```python
from build123d import *

# Parameters (mm, degrees)
F0_W      = 116
F0_H      = 71
F0_W_2    = 70
F0_H_2    = 53
F1_DEPTH  = 2
F2_W      = 116
F2_H      = 71
F2_W_2    = 112
F2_H_2    = 66
F3_DEPTH  = 11
F4_R      = 2.5
F5_R      = 1
F6_R      = 4.5
F6_R_2    = 2
F7_DEPTH  = 5
F8_SIZE   = 1.99999
F9_W      = 15.5
F9_H      = 7.5
F9_W_2    = 26
F9_H_2    = 4
F10_DEPTH = 25
F11_DEPTH = 25


# Not quite as in the source:
# - a fillet or chamfer is up to 0.001 mm smaller than in the source, because OpenCascade refuses the exact size


with BuildPart() as f1:
    # F0 (on Top) → F1 (new body)
    with BuildSketch(Plane.XY):
        with Locations((58, 35.5)):
            Rectangle(F0_W, F0_H)
        with Locations((55, 35.5)):
            Rectangle(F0_W_2, F0_H_2, mode=Mode.SUBTRACT)
    extrude(amount=F1_DEPTH)

    # F2 (on face) → F3 (join)
    with BuildSketch(Plane.XY.offset(2)):
        with Locations((58, 35.5)):
            Rectangle(F2_W, F2_H)
        with Locations((58, 36)):
            Rectangle(F2_W_2, F2_H_2, mode=Mode.SUBTRACT)
    extrude(amount=F3_DEPTH)

    # F4
    f4_edges = [f1.edges().sort_by_distance(p)[0] for p in [
        (0, 0, 6.5),
        (116, 0, 6.5),
        (0, 71, 6.5),
        (116, 71, 6.5),
    ]]
    fillet(f4_edges, radius=F4_R)

    # F5
    f5_edges = [f1.edges().sort_by_distance(p)[0] for p in [
        (114, 3, 7.5),
        (2, 3, 7.5),
        (2, 69, 7.5),
        (114, 69, 7.5),
    ]]
    fillet(f5_edges, radius=F5_R)

    # F6 (on face) → F7 (join)
    with BuildSketch(Plane.XY.offset(2)):
        with Locations((7, 64)):
            Circle(F6_R)
        with Locations((7, 64)):
            Circle(F6_R_2, mode=Mode.SUBTRACT)
        with Locations((7, 8)):
            Circle(F6_R)
        with Locations((7, 8)):
            Circle(F6_R_2, mode=Mode.SUBTRACT)
        with Locations((109, 8)):
            Circle(F6_R)
        with Locations((109, 8)):
            Circle(F6_R_2, mode=Mode.SUBTRACT)
        with Locations((109, 64)):
            Circle(F6_R)
        with Locations((109, 64)):
            Circle(F6_R_2, mode=Mode.SUBTRACT)
    extrude(amount=F7_DEPTH)

    # F8 (size 2 in the source; OpenCascade refuses exactly that, so slightly less here)
    f8_edges = [f1.edges().sort_by_distance(p)[0] for p in [
        (90, 35.5, 0),
        (55, 9, 0),
        (20, 35.5, 0),
        (55, 62, 0),
    ]]
    chamfer(f8_edges, length=F8_SIZE)

    # F9 (on face) → F10 (cut)
    with BuildSketch(Plane(origin=(0, 0, 0), x_dir=(0, -1, 0), z_dir=(-1, 0, 0))):
        with Locations((-54.75, 12.75)):
            Rectangle(F9_W, F9_H)
        with Locations((-26, 11)):
            Rectangle(F9_W_2, F9_H_2)
    extrude(amount=-F10_DEPTH, mode=Mode.SUBTRACT)

    # F11 (cut): faces of the model
    f11_faces = [f1.faces().sort_by_distance(p)[0] for p in [
        (7, 8, 2),
        (7, 64, 2),
        (109, 8, 2),
        (109, 64, 2),
    ]]
    extrude(f11_faces, amount=-F11_DEPTH, mode=Mode.SUBTRACT)


solid = f1.part
```
Verification items for the finished model (mm, model axes). A direction names the side the tool comes from. Coordinates: 2 decimals unless noted, no trailing zeros. Loops run counter-clockwise (first coordinate to the right, second up) from the corner with the lowest first, then second, coordinate; pieces in that order, holes last. Notation, with made-up numbers: (26.25, 72.5) -> (53.25, 72.5) arc R7 cw to (53.25, 83.5) -> close; hole circle Ø5 at (48.5, 76.25). An arc over 180 degrees is marked (long way). Answer in a Markdown table with one row per item. Add a question column.
1. Material ranges on probe 1 along Y at (x, z) = (109, 1.2); probe 2 along Y at (x, z) = (109, 5.9); probe 3 along Y at (x, z) = (64.5, 10), recorded low to high. Write a range as [from, to].
2. Section check B-B, the plane z = 4.75. Give the number of separate pieces and of enclosed holes in the cut face, then the cut area to 3 significant figures.
3. Section check C-C, the plane z = 11.5. Enter the section's corners in (x, y).
4. Draft check along Y on faces 3 (the face through (6.41, 68.46, 4.46)), 4 (the face through (53, 1, 13)), 5 (the face through (57, 0, 6)). Enter one of: +Y half, -Y half, draft (parallel to the pull), parting line (faces both ways), or undercut.
5. Depth check by flat-ended pin: P1, Ø0.6, axis at x = 1, y = 23.5, coming from the +Z side; P2, Ø5, axis at x = 7, y = 64, coming from the +Z side; P3, Ø1.6, axis at x = 1, z = 10.5, coming from the +Y side. Enter the tip coordinate at first touch or a pass-through.
6. Access from +Z, -Z, +X, -X, +Y, -Y to the whole of each face (thin tool, end or side, straight path). Record for faces 1 (the face through (57, 7, 2)), 2 (the face through (0.713, 70.248, 6.409)).
Derived:
| question | item | result |
|---|---|---|
| 1 | probe 1 | y = [0, 6], [10, 62], [66, 71] |
| 1 | probe 2 | y = [0, 3], [3.5, 6], [10, 12.5], [59.5, 62], [66, 68.5], [69, 71] |
| 1 | probe 3 | y = [0, 3], [69, 71] |
| 2 | separate pieces | 5 |
| 2 | enclosed holes | 5 |
| 2 | area | 1,040 mm² |
| 3 | outline | (0, 2.5) arc R2.5 ccw to (2.5, 0) -> (113.5, 0) arc R2.5 ccw to (116, 2.5) -> (116, 68.5) arc R2.5 ccw to (113.5, 71) -> (2.5, 71) arc R2.5 ccw to (0, 68.5) -> (0, 62.5) -> (2, 62.5) -> (2, 68) arc R1 cw to (3, 69) -> (113, 69) arc R1 cw to (114, 68) -> (114, 4) arc R1 cw to (113, 3) -> (3, 3) arc R1 cw to (2, 4) -> (2, 13) -> (0, 13) -> close; (0, 39) -> (2, 39) -> (2, 47) -> (0, 47) -> close |
| 4 | face 3 | undercut |
| 4 | face 4 | draft |
| 4 | face 5 | -Y half |
| 5 | P1 | stops at z = 9 |
| 5 | P2 | stops at z = 7 |
| 5 | P3 | stops at y = 70.9 |
| 6 | face 1 | +Z |
| 6 | face 2 | +Z, -Z, -X, +Y |
